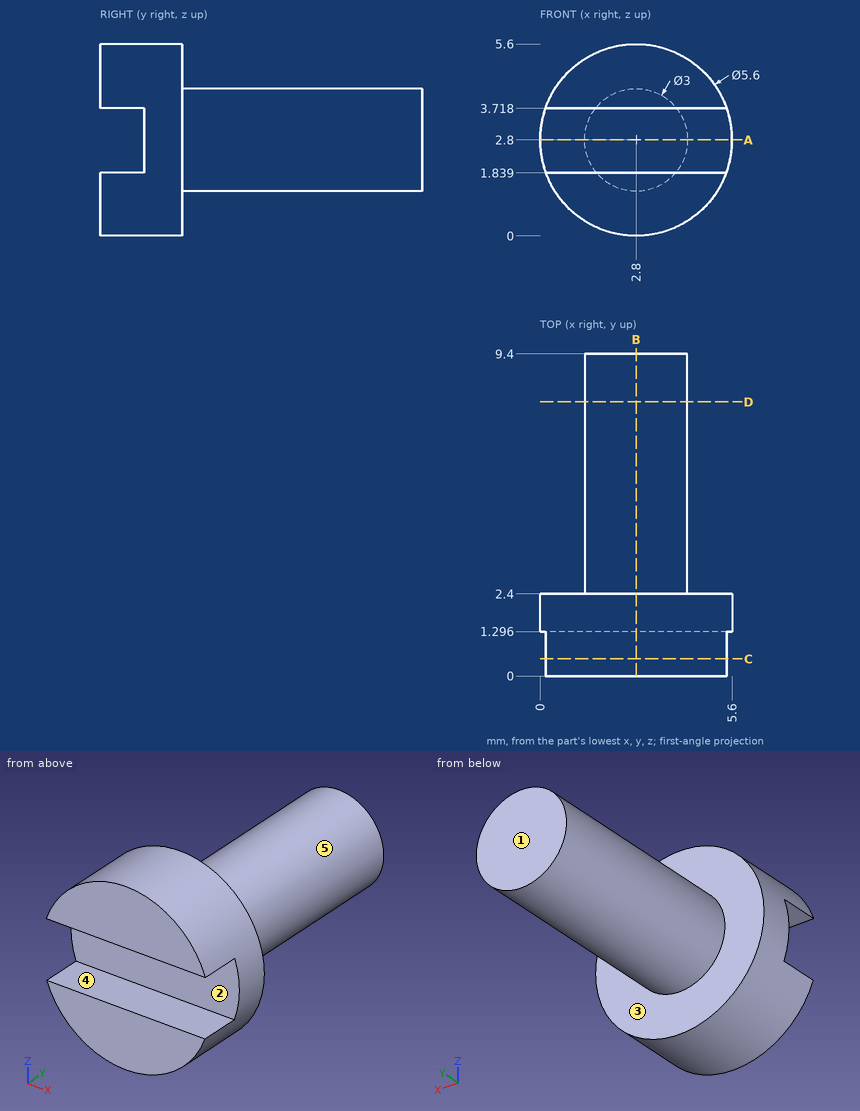
For this review, use the dimensioned drawing (mm, ordinates from the lowest corner) and the shaded views. A direction names the side the tool comes from. Round coordinates to 2 decimals unless told otherwise and drop trailing zeros. Order: outer loops, then holes, each group sorted by start corner. A loop starts at its lowest first (then second) coordinate and runs counter-clockwise, first axis right, second up. Notation, with made-up numbers: (-33.5, 76.5) -> (-14.5, 76.5) arc R19 ccw to (-14.5, 99.5) -> close; hole circle Ø7 at (-13.5, -8). An arc over 180 degrees is marked (long way). One line per item, written item: value. Start each with the question number.
Q1. Take a section at D-D (y = 8). Write out the cut boundary in (x, z).
Q2. Take a section at A-A (z = 2.8). Write out the cut boundary in (x, y), and give its area (3 significant figures).
Q3. Wall thickness on line 1 (Y direction, x = 2.95, z = 2.6); line 2 (Y direction, x = 2.7, z = 5.4); line 3 (Z direction, x = 3.5, y = 1): over which ranges is each line inside the solid? List them lowest first.
Q4. Machinability: for the marked faces 1 and 2, which of the approach directions +Z, -Z, +X, -X, +Y, -Y give a long, thin tool a straight path to every point of the face, cutting with its end or side? Answer none if there is none.
Q5. Clearance check with flat-ended pins moving along their axes: pin 1 Ø3 at (x, y) = (4, 4.5) entering from -Z; pin 2 Ø1.5 at (y, z) = (5.5, 3) entering from -X; pin 3 Ø0.6 at (x, z) = (4, 3) entering from -Y. State where each tip first meets the part, or that it passes through.
Q6. Take a section at B-B (x = 2.8). Write out the cut boundary in (y, z), and give its area (3 significant figures).
Q7. Take a section at C-C (y = 0.5). Write out the cut boundary in (x, z) (1 decimal).
Q8. Mouldability with a two-part tool opening along Z and no side actions: class the marked faces 3, 4 and 5 as released by +Z, released by -Z, zero draft, split by the parting line, or undercut.
Reported:
1. outline: circle Ø3 at (2.8, 2.8)
2. outline: (0, 1.3) -> (5.6, 1.3) -> (5.6, 2.4) -> (4.3, 2.4) -> (4.3, 9.4) -> (1.3, 9.4) -> (1.3, 2.4) -> (0, 2.4) -> close
2. area: 27.2 mm2
3. line 1: y = 1.3 to 9.4
3. line 2: y = 0 to 2.4
3. line 3: z = 0.09 to 1.84, 3.72 to 5.51
4. face 1: +Z, -Z, +X, -X, +Y
4. face 2: +X, -X, -Y
5. pin 1: stops at z = 1.3
5. pin 2: stops at x = 1.3
5. pin 3: stops at y = 1.3
6. outline: (0, 0) -> (2.4, 0) -> (2.4, 1.3) -> (9.4, 1.3) -> (9.4, 4.3) -> (2.4, 4.3) -> (2.4, 5.6) -> (0, 5.6) -> (0, 3.72) -> (1.3, 3.72) -> (1.3, 1.84) -> (0, 1.84) -> close
6. area: 32.0 mm2
7. outline: (0.2, 1.8) arc R2.8 ccw to (5.4, 1.8) -> close; (0.2, 3.7) -> (5.4, 3.7) arc R2.8 ccw to start
8. face 3: zero draft
8. face 4: undercut
8. face 5: split by the parting line
